Model file for the job. Use its own axes, mm. A direction names the side the tool comes from. Give positions to 0.01 mm unless a question says otherwise; leave off trailing zeros. Loops run counter-clockwise (first coordinate to the right, second up) from the corner with the lowest first, then second, coordinate; pieces in that order, holes last. Notation, with made-up numbers: (10, 61) - (17, 61) arc R29 ccw to (17, 94) - close; hole circle Ø7 at (38, -7). An arc over 180 degrees is marked (long way). Use a Markdown table: item, result.
Solid Edge part; units mm, degrees
sketch "Sketch1" plane through (0, 0, 0) normal (0, 0, 1) x (1, 0, 0)
  line L0 (107.2831, 49.8223) -> (107.2831, -121.2368)
  line L1 (107.2831, -121.2368) -> (-89.438, -121.2368)
  line L2 (-89.438, -121.2368) -> (-89.438, 49.8223)
  line L3 (-89.438, 49.8223) -> (107.2831, 49.8223)
  line L4 (-62.5399, 12.7151) -> (-62.5399, 2.7151)
  line L5 (-62.5399, 2.7151) -> (-32.5399, 2.7151)
  line L6 (-32.5399, 2.7151) -> (-32.5399, 12.7151)
  line L7 (-32.5399, 12.7151) -> (-62.5399, 12.7151)
  line L8 (37.4324, -91.4582) -> (37.4324, -101.4582)
  line L9 (37.4324, -101.4582) -> (82.4324, -101.4582)
  line L10 (82.4324, -101.4582) -> (82.4324, -91.4582)
  line L11 (82.4324, -91.4582) -> (37.4324, -91.4582)
  line L12 (27.4324, -43.4085) -> (27.4324, -53.4085)
  line L13 (27.4324, -53.4085) -> (92.4324, -53.4085)
  line L14 (92.4324, -53.4085) -> (92.4324, -43.4085)
  line L15 (92.4324, -43.4085) -> (27.4324, -43.4085)
  line L16 (-70.0676, -43.7069) -> (-70.0676, -53.7069)
  line L17 (-70.0676, -53.7069) -> (-10.0676, -53.7069)
  line L18 (-10.0676, -53.7069) -> (-10.0676, -43.7069)
  line L19 (-10.0676, -43.7069) -> (-70.0676, -43.7069)
  line L20 (-68.4398, -90.3913) -> (-68.4398, -100.3913)
  line L21 (-68.4398, -100.3913) -> (-8.4398, -100.3913)
  line L22 (-8.4398, -100.3913) -> (-8.4398, -90.3913)
  line L23 (-8.4398, -90.3913) -> (-68.4398, -90.3913)
  line L24 (5.3193, 13.0598) -> (5.3193, 3.0598)
  line L25 (5.3193, 3.0598) -> (65.3193, 3.0598)
  line L26 (65.3193, 3.0598) -> (65.3193, 13.0598)
  line L27 (65.3193, 13.0598) -> (5.3193, 13.0598)
  line L28 (33.5794, 40.6994) -> (-16.4206, 40.6994)
  line L29 (-16.4206, 40.6994) -> (-16.4206, 30.6994)
  line L30 (-16.4206, 30.6994) -> (33.5794, 30.6994)
  line L31 (33.5794, 30.6994) -> (33.5794, 40.6994)
  circle A0 centre (53.9449, -6.6083) radius 2.9
  circle A1 centre (-47.5399, -5.9218) radius 3.05
  circle A2 centre (-40.0676, -67.1552) radius 2.55
  circle A3 centre (-40.0676, -110.7563) radius 2.55
  circle A4 centre (59.9324, -110.7563) radius 2.55
  circle A5 centre (59.9324, -67.1552) radius 2.55
  circle A6 centre (16.5449, -25.8083) radius 2.9
  line L32 (51.4449, -23.7083) -> (51.4449, -8.6083)
  line L33 (51.4449, -8.6083) -> (21.1449, -8.6083)
  line L34 (21.1449, -8.6083) -> (21.1449, -23.7083)
  line L35 (21.1449, -23.7083) -> (51.4449, -23.7083)
  circle A7 centre (16.5449, -6.6083) radius 2.9
  circle A8 centre (53.9449, -25.8083) radius 2.9
extrude "Protrusion1" add sketch "Sketch1" along normal blind 2
fillet "Round_1" radius 5 4 edges at (-89.438, -121.2368, 1) (-89.438, 49.8223, 1) (107.2831, -121.2368, 1) (107.2831, 49.8223, 1)
sketch "Sketch2" plane through (0, 0, 0) normal (0, 0, 1) x (1, 0, 0)
  circle A0 centre (-40.0676, -110.7563) radius 4
  circle A1 centre (-40.0676, -110.7563) radius 3
  circle A2 centre (-40.0676, -67.1552) radius 4
  circle A3 centre (-40.0676, -67.1552) radius 3
  circle A4 centre (59.9324, -67.1552) radius 4
  circle A5 centre (59.9324, -67.1552) radius 3
  circle A6 centre (59.9324, -110.7563) radius 4
  circle A7 centre (59.9324, -110.7563) radius 3
extrude "ExtrudedProtrusion_2" add sketch "Sketch2" against normal blind 3
sketch "Sketch3" plane through (8.9225, -35.7072, 2) normal (0, 0, 1) x (1, 0, 0)
  circle A0 centre (-83.9901, -12.9997) radius 1.75
  circle A1 centre (-82.3623, -59.6841) radius 1.75
  circle A2 centre (-12.3623, -59.6841) radius 1.75
  circle A3 centre (-13.9901, -12.9997) radius 1.75
  circle A4 centre (13.5099, -12.9997) radius 2.2946
  circle A5 centre (88.5099, -12.9997) radius 1.75
  circle A6 centre (78.5099, -60.751) radius 1.75
  circle A7 centre (23.5099, -60.751) radius 1.75
  circle A8 centre (61.3967, 43.767) radius 1.75
  circle A9 centre (-8.6033, 43.767) radius 1.75
  circle A10 centre (29.6569, 71.4066) radius 1.75
  circle A11 centre (-30.3431, 71.4066) radius 1.75
  circle A12 centre (-36.4625, 43.767) radius 1.75
  circle A13 centre (-76.4625, 43.767) radius 1.75
extrude "ExtrudedCutout_1" cut sketch "Sketch3" against normal blind 56
sketch "Sketch4" plane through (0, 0, 0) normal (0, 0, 1) x (1, 0, 0)
  circle A0 centre (16.5449, -25.8083) radius 2.9
  circle A1 centre (16.5449, -6.6083) radius 2.9
  circle A2 centre (53.9449, -6.6083) radius 2.9
  circle A3 centre (53.9449, -25.8083) radius 2.9
extrude "ExtrudedProtrusion_4" add sketch "Sketch4" along normal blind 2
sketch "Sketch5" plane through (0, 0, 0) normal (0, 0, 1) x (1, 0, 0)
  circle A0 centre (16.5449, -25.8083) radius 2.9
  circle A1 centre (16.5449, -25.8083) radius 1.45
  circle A2 centre (16.5449, -6.6083) radius 2.9
  circle A3 centre (16.5449, -6.6083) radius 1.45
  circle A4 centre (53.9449, -6.6083) radius 2.9
  circle A5 centre (53.9449, -6.6083) radius 1.45
  circle A6 centre (53.9449, -25.8083) radius 2.9
  circle A7 centre (53.9449, -25.8083) radius 1.45
extrude "ExtrudedProtrusion_5" add sketch "Sketch5" against normal blind 6
(1) 3-axis set-ups, long thin cutter, end or side, ignore diameter. For faces 5 (the cylindrical face through (61.3, -112.91, 0.99)), 6 (the cylindrical face through (-38.683, -113.418, -1.479)): which of +Z, -Z, +X, -X, +Y, -Y reach the whole face in a straight line?
Computed:
| item | result |
|---|---|
| face 5 | +Z, -Z |
| face 6 | -Z |
(2) Slice it at A-A, the plane x = -56. Write the cut outline in (y, z).
Computed:
| item | result |
|---|---|
| outline | (-121.24, 0) - (-100.39, 0) - (-100.39, 2) - (-121.24, 2) - close; (-90.39, 0) - (-53.71, 0) - (-53.71, 2) - (-90.39, 2) - close; (-43.71, 0) - (2.72, 0) - (2.72, 2) - (-43.71, 2) - close; (12.72, 0) - (49.82, 0) - (49.82, 2) - (12.72, 2) - close |
(3) Slice it at D-D, the plane y = -59. Write the cut outline in (x, z), plus the area to 3 significant figures.
Computed:
| item | result |
|---|---|
| outline | (-89.44, 0) - (107.28, 0) - (107.28, 2) - (-89.44, 2) - close |
| area | 393 mm² |
(4) Pin check, flat tips, straight feed: P1, Ø5, axis at x = 83, y = 32.5, coming from the -Z side; P2, Ø4.5, axis at x = -21.42, y = 35.7, coming from the +Z side; P3, Ø2.5, axis at x = -38.5, y = -109.5, coming from the -Z side. Stop position of each tip, or through.
Computed:
| item | result |
|---|---|
| P1 | z = 0 |
| P2 | z = 2 |
| P3 | z = -3 |
(5) Slice it at B-B, the plane y = -17.5. Write the cut outline in (x, z).
Computed:
| item | result |
|---|---|
| outline | (-89.44, 0) - (21.14, 0) - (21.14, 2) - (-89.44, 2) - close; (51.44, 0) - (107.28, 0) - (107.28, 2) - (51.44, 2) - close |
(6) Slice it at C-C, the plane z = -4.75. Write the cut outline in (x, y).
Computed:
| item | result |
|---|---|
| outline | circle Ø5.8 at (16.54, -25.81); circle Ø5.8 at (16.54, -6.61); circle Ø5.8 at (53.94, -25.81); circle Ø5.8 at (53.94, -6.61); hole circle Ø2.9 at (16.54, -25.81); hole circle Ø2.9 at (16.54, -6.61); hole circle Ø2.9 at (53.94, -25.81); hole circle Ø2.9 at (53.94, -6.61) |
(7) Drill centre lines: probe 1 along Y at (x, z) = (36, 1); probe 2 along X at (y, z) = (5.5, 0.25); probe 3 along Z at (x, y) = (-59, -62). Where is each one in solid material? Low to high. Write a range as [from, to].
Computed:
| item | result |
|---|---|
| probe 1 | [-121.24, -53.41], [-43.41, -23.71], [-8.61, 3.06], [13.06, 49.82] |
| probe 2 | [-89.44, -62.54], [-32.54, 5.32], [65.32, 107.28] |
| probe 3 | [0, 2] |
(8) Mould opens along X. For faces 1 (the flat face through (-39, -64, -3)), 2 (the flat face through (-38, -109, 0)), 3 (the cylindrical face through (105.857, 48.319, 1.014)), 4 (the cylindrical face through (62.794, -66.254, -1.479)) say: pulls with the +X half, pulls with the -X half, needs draft (parallel to the pull), parting line crosses it, or undercut.
Computed:
| item | result |
|---|---|
| face 1 | needs draft |
| face 2 | undercut |
| face 3 | pulls with the +X half |
| face 4 | undercut |
